from build123d import *

# Parameters (mm, degrees)
SK_P01_PACK_W   = 90
SK_P01_PACK_H   = 75
P01_PACK_DEPTH  = 42
P02_STRAP_START = 42
SK_P02_STRAP_W  = 18
SK_P02_STRAP_H  = 77
P02_STRAP_DEPTH = 1.5
P03_STRAP_START = 42
SK_P03_STRAP_W  = 18
SK_P03_STRAP_H  = 77
P03_STRAP_DEPTH = 1.5
SK_P04_STRAP_W  = 14
SK_P04_STRAP_H  = 2
P04_STRAP_DEPTH = 42
SK_P05_STRAP_W  = 14
SK_P05_STRAP_H  = 2
P05_STRAP_DEPTH = 42
SK_P06_STRAP_W  = 14
SK_P06_STRAP_H  = 2
P06_STRAP_DEPTH = 42
SK_P07_STRAP_W  = 14
SK_P07_STRAP_H  = 2
P07_STRAP_DEPTH = 42


with BuildPart() as part:
    # SK_P01_Pack → P01_Pack (new body)
    with BuildSketch(Plane(origin=(0, 0, 0), x_dir=(1, 0, 0), z_dir=(0, 1, 0))):
        Rectangle(SK_P01_PACK_W, SK_P01_PACK_H)
    extrude(amount=P01_PACK_DEPTH)

    # SK_P02_Strap → P02_Strap (add)
    with BuildSketch(Plane(origin=(0, 0, 0), x_dir=(1, 0, 0), z_dir=(0, 1, 0)).offset(P02_STRAP_START)):
        with Locations((-22.5, 0)):
            Rectangle(SK_P02_STRAP_W, SK_P02_STRAP_H)
    extrude(amount=P02_STRAP_DEPTH)

    # SK_P03_Strap → P03_Strap (add)
    with BuildSketch(Plane(origin=(0, 0, 0), x_dir=(1, 0, 0), z_dir=(0, 1, 0)).offset(P03_STRAP_START)):
        with Locations((22.5, 0)):
            Rectangle(SK_P03_STRAP_W, SK_P03_STRAP_H)
    extrude(amount=P03_STRAP_DEPTH)

    # SK_P04_Strap → P04_Strap (add)
    with BuildSketch(Plane(origin=(0, 0, 0), x_dir=(1, 0, 0), z_dir=(0, 1, 0))):
        with Locations((-22.5, 38.5)):
            Rectangle(SK_P04_STRAP_W, SK_P04_STRAP_H)
    extrude(amount=P04_STRAP_DEPTH)

    # SK_P05_Strap → P05_Strap (add)
    with BuildSketch(Plane(origin=(0, 0, 0), x_dir=(1, 0, 0), z_dir=(0, 1, 0))):
        with Locations((-22.5, -38.5)):
            Rectangle(SK_P05_STRAP_W, SK_P05_STRAP_H)
    extrude(amount=P05_STRAP_DEPTH)

    # SK_P06_Strap → P06_Strap (add)
    with BuildSketch(Plane(origin=(0, 0, 0), x_dir=(1, 0, 0), z_dir=(0, 1, 0))):
        with Locations((22.5, 38.5)):
            Rectangle(SK_P06_STRAP_W, SK_P06_STRAP_H)
    extrude(amount=P06_STRAP_DEPTH)

    # SK_P07_Strap → P07_Strap (add)
    with BuildSketch(Plane(origin=(0, 0, 0), x_dir=(1, 0, 0), z_dir=(0, 1, 0))):
        with Locations((22.5, -38.5)):
            Rectangle(SK_P07_STRAP_W, SK_P07_STRAP_H)
    extrude(amount=P07_STRAP_DEPTH)


solid = part.part
Verification items for the finished model (mm, model axes). A direction names the side the tool comes from. Give positions to 0.01 mm unless a question says otherwise; leave off trailing zeros. Write each loop counter-clockwise with the first axis right and the second up, starting at its lowest first coordinate (ties: lowest second). Pieces come first, ordered by that corner, then holes. Notation, with made-up numbers: (-7, 71) -> (45, 71) arc R27 cw to (45, 100) -> close; hole circle Ø5 at (-38, 62). An arc over 180 degrees is marked (long way). Use CSV: the item, a comma, the result in double quotes.
(1) Sectioned sample at B-B (z = 30.5). Record the cut outline in (x, y), plus the area to 3 significant figures.
Derived:
outline,"(-45, 0) -> (45, 0) -> (45, 42) -> (31.5, 42) -> (31.5, 43.5) -> (13.5, 43.5) -> (13.5, 42) -> (-13.5, 42) -> (-13.5, 43.5) -> (-31.5, 43.5) -> (-31.5, 42) -> (-45, 42) -> close"
area,"3,830 mm^2"
(2) Go/stop test with flat-tipped pins: pin 1 (5 mm diameter, centred on x = 7, y = 29, fed in from +Z); pin 2 (0.8 mm diameter, centred on x = -19, y = 42.5, fed in from -Z); pin 3 (5 mm diameter, centred on x = -33.5, z = -26, fed in from -Y); pin 4 (1.6 mm diameter, centred on y = 17.5, z = -39, fed in from +X). Record where each tip stops, or that it passes through.
Derived:
pin 1,"stops at z = 37.5"
pin 2,"stops at z = -38.5"
pin 3,"stops at y = 0"
pin 4,"stops at x = 29.5"
(3) Release check for a two-part mould opening along X. For faces 1 (the flat face through (45, 21, 1)), 2 (the flat face through (-23, 21, 39.5)), 3 (the flat face through (-29.5, 21, 39)), 4 (the flat face through (15.5, 21, 39)) record: +X half, -X half, draft (parallel to the pull), parting line (faces both ways), or undercut.
Derived:
face 1,"+X half"
face 2,"draft"
face 3,"-X half"
face 4,"undercut"
(4) Sectioned sample at C-C (x = 34.5). Record the cut outline in (y, z), plus the area to 3 significant figures.
Derived:
outline,"(0, -37.5) -> (42, -37.5) -> (42, 37.5) -> (0, 37.5) -> close"
area,"3,150 mm^2"
(5) Set-up check for faces 5 (the flat face through (29.5, 21, -38)), 6 (the flat face through (-15.5, 21, 39)), 7 (the flat face through (-29.5, 21, -38)): record each of +Z, -Z, +X, -X, +Y, -Y from which the full face is reachable in a straight line by a thin tool's end or side.
Derived:
face 5,"-Z, +X, -Y"
face 6,"+Z, -Y"
face 7,"-Z, -X, -Y"
(6) Sectioned sample at A-A (y = 33.5). Record the cut outline in (x, z).
Derived:
outline,"(-45, -37.5) -> (-29.5, -37.5) -> (-29.5, -39.5) -> (-15.5, -39.5) -> (-15.5, -37.5) -> (15.5, -37.5) -> (15.5, -39.5) -> (29.5, -39.5) -> (29.5, -37.5) -> (45, -37.5) -> (45, 37.5) -> (29.5, 37.5) -> (29.5, 39.5) -> (15.5, 39.5) -> (15.5, 37.5) -> (-15.5, 37.5) -> (-15.5, 39.5) -> (-29.5, 39.5) -> (-29.5, 37.5) -> (-45, 37.5) -> close"
(7) Material ranges on L1, parallel to Z at x = -34, y = 7; L2, parallel to Y at x = -10, z = -15.5, recorded low to high.
Derived:
L1,"z = -37.5 to 37.5"
L2,"y = 0 to 42"
